Input: part model. Units: mm. Frame: model coordinates. A direction names the side the tool comes from. Coordinates: 2 decimals unless noted, no trailing zeros. Loops run counter-clockwise (first coordinate to the right, second up) from the corner with the lowest first, then second, coordinate; pieces in that order, holes last. Notation, with made-up numbers: (-35.5, -8) -> (5.5, -8) arc R20 cw to (5.5, 14) -> close; hole circle Ø6 at (60, -17). An arc over 180 degrees is marked (long way). Answer as a JSON object with one key per item and string values.
Autodesk Inventor part; units mm, degrees
ref_plane "BODY_N_XY" through (197, 0, 0) normal (0, 0, -1) x (1, 0, 0)
ref_plane "BODY_N_YZ" through (197, 0, 0) normal (1, 0, 0) x (0, -1, 0)
ref_plane "BODY_N_ZX" through (197, 0, 0) normal (0, -1, 0) x (0, 0, -1)
sketch "Sketch_8" plane through (0, 0, 0) normal (0, 0, 1) x (1, 0, 0)
  line L0 (0, 0) -> (-8, 0)
  line L1 (-8, 0) -> (-8, 4.3865)
  line L2 (-8, 4.3865) -> (-7.3865, 5)
  line L3 (-7.3865, 5) -> (0, 5)
  line L4 (0, 5) -> (0, 0)
  line L5 (0, 0) -> (-8, 0)
revolve "Revolution1" add sketch "Sketch_8" angle 360 about axis through (0, 0, 0) along (1, 0, 0)
thread "Thread1"
sketch "Sketch_9" plane through (0, 0, 0) normal (1, 0, 0) x (0, 0, -1)
  line L0 (-9.15, 4.0345) -> (-9.15, -4.0345)
  arc A0 (-9.15, -4.0345) -> (-4.0345, -9.15) centre (0, 0) ccw
  line L1 (-4.0345, -9.15) -> (4.0345, -9.15)
  arc A1 (4.0345, -9.15) -> (9.15, -4.0345) centre (0, 0) ccw
  line L2 (9.15, -4.0345) -> (9.15, 4.0345)
  arc A2 (9.15, 4.0345) -> (4.0345, 9.15) centre (0, 0) ccw
  line L3 (4.0345, 9.15) -> (-4.0345, 9.15)
  arc A3 (-4.0345, 9.15) -> (-9.15, 4.0345) centre (0, 0) ccw
extrude "Extrusion1" add sketch "Sketch_9" along normal blind 12.5
sketch "Sketch_11" plane through (12.5, 0, 0) normal (1, 0, 0) x (0, 0, -1)
  circle A0 centre (0, 0) radius 8.7
extrude "Extrusion2" add sketch "Sketch_11" along normal blind 175
sketch "Sketch_10" plane through (187.5, 0, 0) normal (1, 0, 0) x (0, 0, -1)
  line L0 (-9.15, 4.0345) -> (-9.15, -4.0345)
  arc A0 (-9.15, -4.0345) -> (-4.0345, -9.15) centre (0, 0) ccw
  line L1 (-4.0345, -9.15) -> (4.0345, -9.15)
  arc A1 (4.0345, -9.15) -> (9.15, -4.0345) centre (0, 0) ccw
  line L2 (9.15, -4.0345) -> (9.15, 4.0345)
  arc A2 (9.15, 4.0345) -> (4.0345, 9.15) centre (0, 0) ccw
  line L3 (4.0345, 9.15) -> (-4.0345, 9.15)
  arc A3 (-4.0345, 9.15) -> (-9.15, 4.0345) centre (0, 0) ccw
extrude "Extrusion3" add sketch "Sketch_10" along normal blind 9.5
sketch "Sketch7" plane through (0, 0, 0) normal (0, 0, 1) x (1, 0, 0)
  line L0 (8, 9.15) -> (8, 4.15)
  line L1 (8, 2.9566) -> (5.933, 4.15)
  line L2 (5.933, 4.15) -> (5.933, 8.717)
  line L3 (5.933, 8.717) -> (5.5, 9.15)
  line L4 (5.5, 9.15) -> (8, 9.15)
  line L5 (8, 9.15) -> (8, 2.9566)
revolve "Revolution2" cut sketch "Sketch7" angle 360 about axis through (8, 9.15, 0) along (0, 1, 0)
thread "Thread2"
sketch "Sketch_7" plane through (0, 0, 0) normal (0, 0, 1) x (1, 0, 0)
  line L0 (192, 9.15) -> (192, 4.15)
  line L1 (192, 2.9566) -> (189.933, 4.15)
  line L2 (189.933, 4.15) -> (189.933, 8.717)
  line L3 (189.933, 8.717) -> (189.5, 9.15)
  line L4 (189.5, 9.15) -> (192, 9.15)
  line L5 (192, 9.15) -> (192, 2.9566)
revolve "Revolution3" cut sketch "Sketch_7" angle 360 about axis through (192, 9.15, 0) along (0, 1, 0)
thread "Thread3"
sketch "Sketch_16" plane through (0, 0, 0) normal (0, 0, 1) x (1, 0, 0)
  line L0 (167.5, 0) -> (-8, 0)
  line L1 (-8, 0) -> (-8, 2.5)
  line L2 (-8, 2.5) -> (12.5, 2.5)
  line L3 (12.5, 2.5) -> (12.5, 8)
  line L4 (12.5, 8) -> (167.5, 8)
  line L5 (167.5, 8) -> (167.5, 0)
  line L6 (167.5, 0) -> (-8, 0)
revolve "Revolution4" cut sketch "Sketch_16" angle 360 about axis through (167.5, 0, 0) along (1, 0, 0)
ref_plane "BODY_N_XY" through (197, 0, 0) normal (0, 0, -1) x (1, 0, 0)
ref_plane "BODY_N_YZ" through (197, 0, 0) normal (1, 0, 0) x (0, -1, 0)
ref_plane "BODY_N_ZX" through (197, 0, 0) normal (0, -1, 0) x (0, 0, -1)
ref_plane "NUT2_XY" through (197, 0, 0) normal (1, 0, 0) x (0, 0, -1)
ref_plane "NUT2_YZ" through (197, 0, 0) normal (0, 0, -1) x (0, 1, 0)
ref_plane "NUT2_ZX" through (197, 0, 0) normal (0, 1, 0) x (1, 0, 0)
ref_plane "SW1_XY" through (17.5, 0, 0) normal (1, 0, 0) x (0, 0, -1)
ref_plane "SW1_YZ" through (17.5, 0, 0) normal (0, 0, -1) x (0, 1, 0)
ref_plane "SW1_ZX" through (17.5, 0, 0) normal (0, 1, 0) x (1, 0, 0)
ref_plane "SW2_XY" through (182.5, 0, 0) normal (-1, 0, 0) x (0, 0, -1)
ref_plane "SW2_YZ" through (182.5, 0, 0) normal (0, 0, -1) x (0, -1, 0)
ref_plane "SW2_ZX" through (182.5, 0, 0) normal (0, -1, 0) x (-1, 0, 0)
ref_plane "SW_R1_XY" through (17.5, -14.15, 0) normal (1, 0, 0) x (0, 0, -1)
ref_plane "SW_R1_YZ" through (17.5, -14.15, 0) normal (0, 0, -1) x (0, 1, 0)
ref_plane "SW_R1_ZX" through (17.5, -14.15, 0) normal (0, 1, 0) x (1, 0, 0)
ref_plane "SW_R2_XY" through (182.5, -14.15, 0) normal (-1, 0, 0) x (0, 0, -1)
ref_plane "SW_R2_YZ" through (182.5, -14.15, 0) normal (0, 0, -1) x (0, -1, 0)
ref_plane "SW_R2_ZX" through (182.5, -14.15, 0) normal (0, -1, 0) x (-1, 0, 0)
ref_plane "body_XY" through (0, 0, 0) normal (1, 0, 0) x (0, 0, -1)
ref_plane "body_YZ" through (0, 0, 0) normal (0, 0, -1) x (0, 1, 0)
ref_plane "body_ZX" through (0, 0, 0) normal (0, 1, 0) x (1, 0, 0)
properties part number "CJ2B16-150Z(1_0)_BODY"
1. Pin query (flat end, axial travel): P1, Ø6, axis at x = 173, z = -5, coming from the -Y side; P2, Ø1.5, axis at x = 81, y = 3, coming from the +Z side; P3, Ø5, axis at x = 154.5, z = -4, coming from the +Y side. Return the tip coordinate at first contact, or that it passes through.
Reply:
{"P1": "stops at y = -8.47", "P2": "stops at z = 8.4", "P3": "stops at y = 8.57"}
2. Section query B-B (x = 115). Return loops of the section in (y, z), plus the area to 3 significant figures.
Reply:
{"outline": "circle Ø17.4 at (0, 0); hole circle Ø16 at (0, 0)", "area": "36.7 mm2"}
3. Section query A-A (y = 0). Return loops of the section in (x, z), plus the area to 3 significant figures.
Reply:
{"outline": "(-8, -4.39) -> (-7.39, -5) -> (0, -5) -> (0, -9.15) -> (12.5, -9.15) -> (12.5, -8.7) -> (187.5, -8.7) -> (187.5, -9.15) -> (197, -9.15) -> (197, 9.15) -> (187.5, 9.15) -> (187.5, 8.7) -> (12.5, 8.7) -> (12.5, 9.15) -> (0, 9.15) -> (0, 5) -> (-7.39, 5) -> (-8, 4.39) -> (-8, 2.5) -> (12.5, 2.5) -> (12.5, 8) -> (167.5, 8) -> (167.5, -8) -> (12.5, -8) -> (12.5, -2.5) -> (-8, -2.5) -> close", "area": "945 mm2"}
4. Access query for faces 4 (the face through (-8, 2, -2)), 5 (the face through (0, -4, -4)), 6 (the face through (98.775, 8.493, 1.886)). Directions: +Z, -Z, +X, -X, +Y, -Y. A direction counts if a zero-diameter tool reaches every point of the face in a straight line with its end or side. Return the directions, or none.
Reply:
{"face 4": "+Z, -Z, -X, +Y, -Y", "face 5": "-X", "face 6": "none"}
5. Line query: line 1 along X through (y, z) = (5.25, 8.25); line 2 along X through (y, z) = (1.75, -2.25); line 3 along X through (y, z) = (8.25, -0.5). Output: solid intervals per line, ascending.
Reply:
{"line 1": "x = 0 to 12.5, 187.5 to 197", "line 2": "x = -8 to 12.5, 167.5 to 197", "line 3": "x = 0 to 5.99, 10.01 to 189.99, 194.01 to 197"}
6. Mould query, pull axis Z, two halves, no side actions, for faces 1 (the face through (2.39, -0.54, -2.44)), 2 (the face through (6, -9.15, 0)), 3 (the face through (192.18, -7.03, -7.11)). Classes: pulls with the +Z half, pulls with the -Z half, needs draft (parallel to the pull), parting line crosses it, or undercut.
Reply:
{"face 1": "undercut", "face 2": "needs draft", "face 3": "pulls with the -Z half"}
